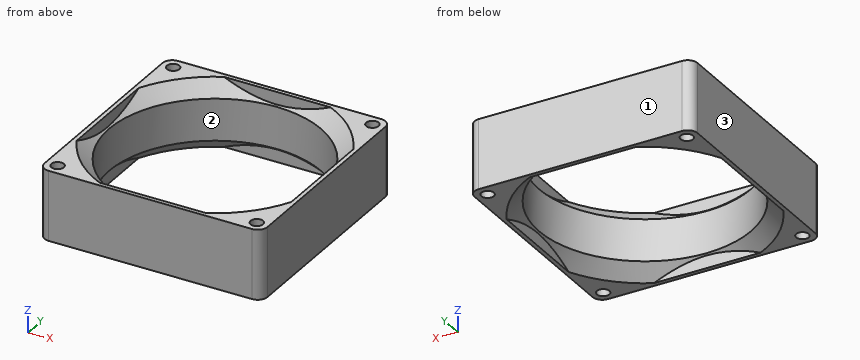
from build123d import *

# Parameters (mm, degrees)
F0_R     = 2.25
F0_R_2   = 38
F1_DEPTH = 25
F3_W     = 1.5
F3_H     = 38.3014360044
F3_W_2   = 38.3014360044
F3_H_2   = 1.5
F4_DEPTH = 25


# Not quite as in the source:
# - a fillet or chamfer that OpenCascade refuses, or shapes differently, is made with other operations: its cross-section is extruded or revolved along the edge and cut away or added


with BuildPart() as f1:
    # F0 (on Top) → F1 (new body)
    with BuildSketch(Plane.XY):
        with BuildLine():
            Line((-36.5, -40), (36.5, -40))
            ThreePointArc((36.5, -40), (38.9748737342, -38.9748737342), (40, -36.5))
            Line((40, -36.5), (40, 36.5))
            ThreePointArc((40, 36.5), (38.9748737342, 38.9748737342), (36.5, 40))
            Line((36.5, 40), (-36.5, 40))
            ThreePointArc((-36.5, 40), (-38.9748737342, 38.9748737342), (-40, 36.5))
            Line((-40, 36.5), (-40, -36.5))
            ThreePointArc((-40, -36.5), (-38.9748737342, -38.9748737342), (-36.5, -40))
        make_face()
        with Locations((-35.75, -35.75)):
            Circle(F0_R, mode=Mode.SUBTRACT)
        with Locations((35.75, -35.75)):
            Circle(F0_R, mode=Mode.SUBTRACT)
        with Locations((-35.75, 35.75)):
            Circle(F0_R, mode=Mode.SUBTRACT)
        Circle(F0_R_2, mode=Mode.SUBTRACT)
        with Locations((35.75, 35.75)):
            Circle(F0_R, mode=Mode.SUBTRACT)
    extrude(amount=F1_DEPTH)

    # F2: chamfer of 5 on 2 edges, made by hand

    # F2_s1 → F2_t2 (revolve, cut)
    with BuildSketch(Plane.XZ):
        Polygon((38, 20), (43, 25), (38, 25), align=None)
    revolve(axis=Axis((0, 0, 25), (0, 0, 1)), mode=Mode.SUBTRACT)

    # F2_s3 → F2_t4 (revolve, cut)
    with BuildSketch(Plane.XZ):
        Polygon((38, 5), (43, 0), (38, 0), align=None)
    revolve(axis=Axis((0, 0, 0), (0, 0, 1)), mode=Mode.SUBTRACT)

    # F3 (on face) → F4 (join, through all)
    with BuildSketch(Plane.XY.offset(25)):
        with Locations((-39.25, 0)):
            Rectangle(F3_W, F3_H)
        with Locations((0, -39.25)):
            Rectangle(F3_W_2, F3_H_2)
        with Locations((39.25, 0)):
            Rectangle(F3_W, F3_H)
        with Locations((0, 39.25)):
            Rectangle(F3_W_2, F3_H_2)
    extrude(amount=-F4_DEPTH)


solid = f1.part
Could you check a few things on this model? Use its own coordinates, in mm. Face numbers are marked on the shaded views. Give positions to 0.01 mm unless a question says otherwise; leave off trailing zeros. Write each loop counter-clockwise with the first axis right and the second up, starting at its lowest first coordinate (ties: lowest second). Pieces come first, ordered by that corner, then holes. Notation, with made-up numbers: (-19.75, 30) -> (-2.75, 30) arc R36 ccw to (-2.75, 65) -> close; hole circle Ø5 at (50.25, 63). An arc over 180 degrees is marked (long way). Answer as a JSON object with one key per item and string values.
Q1. Will these pins go through, and if not, where does the flat tip stop? pin 1 Ø5 at (x, y) = (31.5, 18.5) entering from +Z; pin 2 Ø5 at (x, y) = (-35.75, -35.75) entering from +Z.
Taken from the geometry:
{"pin 1": "stops at z = 21.03", "pin 2": "stops at z = 25"}
Q2. Please list where these lines run through material, in increasing order: L1, parallel to X at y = -8, z = 22.25; L2, parallel to Y at x = 0, z = 15.5; L3, parallel to X at y = -35, z = 15.5.
Taken from the geometry:
{"L1": "x = -40 to -38.5, 38.5 to 40", "L2": "y = -40 to -38, 38 to 40", "L3": "x = -40 to -37.87, -33.63 to -14.8, 14.8 to 33.63, 37.87 to 40"}
Q3. Suppose I cut it at C-C on z = 6.25. Write out the boundary of the cut face in (x, y).
Taken from the geometry:
{"outline": "(-40, -36.5) arc R3.5 ccw to (-36.5, -40) -> (36.5, -40) arc R3.5 ccw to (40, -36.5) -> (40, 36.5) arc R3.5 ccw to (36.5, 40) -> (-36.5, 40) arc R3.5 ccw to (-40, 36.5) -> close; hole circle Ø4.5 at (-35.75, -35.75); hole circle Ø76 at (0, 0); hole circle Ø4.5 at (-35.75, 35.75); hole circle Ø4.5 at (35.75, -35.75); hole circle Ø4.5 at (35.75, 35.75)"}
Q4. We'd pull the mould along Y, two halves only. Please class the marked faces 1, 2 and 3: released by +Y, released by -Y, zero draft, split by the parting line, or undercut.
Taken from the geometry:
{"face 1": "released by +Y", "face 2": "undercut", "face 3": "zero draft"}
Q5. Suppose I cut it at A-A on x = 0. Write out the boundary of the cut face in (y, z).
Taken from the geometry:
{"outline": "(-40, 0) -> (-38.5, 0) -> (-38.5, 4.5) -> (-38, 5) -> (-38, 20) -> (-38.5, 20.5) -> (-38.5, 25) -> (-40, 25) -> close; (38, 5) -> (38.5, 4.5) -> (38.5, 0) -> (40, 0) -> (40, 25) -> (38.5, 25) -> (38.5, 20.5) -> (38, 20) -> close"}
